from build123d import *

# Parameters (mm, degrees)
SKETCH1_W           = 40.8
SKETCH1_H           = 20
BOSS_EXTRUDE1_DEPTH = 36.4
SKETCH2_W           = 40.8
SKETCH2_H           = 20
SKETCH2_W_2         = 37.24847256
SKETCH2_H_2         = 17
CUT_EXTRUDE1_DEPTH  = 4.6
SKETCH3_W           = 37.24847256
SKETCH3_H           = 17
SKETCH3_R           = 5
CUT_EXTRUDE2_DEPTH  = 3.9
SKETCH4_R           = 5
SKETCH4_R_2         = 3.5
CUT_EXTRUDE3_DEPTH  = 3
FILLET1_R           = 1
FILLET2_R           = 0.25


with BuildPart() as part:
    # Sketch1 → Boss-Extrude1 (new body)
    with BuildSketch(Plane(origin=(0, 0, 0), x_dir=(1, 0, 0), z_dir=(0, 1, 0))):
        Rectangle(SKETCH1_W, SKETCH1_H)
    extrude(amount=BOSS_EXTRUDE1_DEPTH)

    # Sketch2 → Cut-Extrude1 (cut)
    with BuildSketch(Plane(origin=(0, 0, 0), x_dir=(1, 0, 0), z_dir=(0, 1, 0))):
        Rectangle(SKETCH2_W, SKETCH2_H)
        Rectangle(SKETCH2_W_2, SKETCH2_H_2, mode=Mode.SUBTRACT)
    extrude(amount=CUT_EXTRUDE1_DEPTH, mode=Mode.SUBTRACT)

    # Sketch3 → Cut-Extrude2 (cut)
    with BuildSketch(Plane(origin=(0, 0, 0), x_dir=(1, 0, 0), z_dir=(0, 1, 0))):
        Rectangle(SKETCH3_W, SKETCH3_H)
        with Locations((9.31211814, 0)):
            Circle(SKETCH3_R, mode=Mode.SUBTRACT)
    extrude(amount=CUT_EXTRUDE2_DEPTH, mode=Mode.SUBTRACT)

    # Sketch4 → Cut-Extrude3 (cut)
    with BuildSketch(Plane(origin=(0, 0, 0), x_dir=(1, 0, 0), z_dir=(0, 1, 0))):
        with Locations((9.31211814, 0)):
            Circle(SKETCH4_R)
        with Locations((9.31211814, 0)):
            Circle(SKETCH4_R_2, mode=Mode.SUBTRACT)
    extrude(amount=CUT_EXTRUDE3_DEPTH, mode=Mode.SUBTRACT)

    # Fillet1
    fillet1_edges = [part.edges().sort_by_distance(p)[0] for p in [
        (20.4, 36.4, 0),
        (0, 36.4, -10),
        (-20.4, 4.6, 0),
        (0, 4.6, 10),
        (20.4, 4.6, 0),
        (0, 4.6, -10),
        (-20.4, 36.4, 0),
        (0, 36.4, 10),
        (-20.4, 20.5, -10),
        (20.4, 20.5, -10),
        (20.4, 20.5, 10),
        (-20.4, 20.5, 10),
    ]]
    fillet(fillet1_edges, radius=FILLET1_R)

    # Fillet2
    fillet2_edges = [part.edges().sort_by_distance(p)[0] for p in [
        (-18.62423628, 4.6, 0),
        (0, 4.6, 8.5),
        (18.62423628, 4.6, 0),
        (18.62423628, 4.25, -8.5),
        (0, 4.6, -8.5),
        (-18.62423628, 4.25, -8.5),
        (-18.62423628, 3.9, 0),
        (0, 3.9, 8.5),
        (18.62423628, 3.9, 0),
        (0, 3.9, -8.5),
    ]]
    fillet(fillet2_edges, radius=FILLET2_R)


solid = part.part
Here's how the part is built. I have some questions about the finished solid (model axes, mm). A direction names the side the tool comes from. Round coordinates to 2 decimals unless told otherwise and drop trailing zeros. Loops run counter-clockwise (first coordinate to the right, second up) from the corner with the lowest first, then second, coordinate; pieces in that order, holes last.
1. If I drill on line 1 along Y through (x, z) = (-5.5, 2.5); line 2 along Z through (x, y) = (10, 35.5); line 3 along Y through (x, z) = (-17, 9.25), over which ranges is the centre line in solid material (lowest first)?
Answer list:
line 1: y = 3.9 to 36.4
line 2: z = -9.99 to 9.99
line 3: y = 4.63 to 36.37
2. If we section it at A-A on z = 0: Write out the boundary of the cut face in (x, y), plus the area to 3 significant figures.
Answer list:
outline: (-20.4, 5.6) arc R1 ccw to (-19.4, 4.6) - (-18.87, 4.6) arc R0.25 cw to (-18.62, 4.35) - (-18.62, 4.15) arc R0.25 ccw to (-18.37, 3.9) - (4.31, 3.9) - (4.31, 3) - (5.81, 3) - (5.81, 0) - (12.81, 0) - (12.81, 3) - (14.31, 3) - (14.31, 3.9) - (18.37, 3.9) arc R0.25 ccw to (18.62, 4.15) - (18.62, 4.35) arc R0.25 cw to (18.87, 4.6) - (19.4, 4.6) arc R1 ccw to (20.4, 5.6) - (20.4, 35.4) arc R1 ccw to (19.4, 36.4) - (-19.4, 36.4) arc R1 ccw to (-20.4, 35.4) - close
area: 1,350 mm2
3. For P1, Ø5.5, axis at x = -3.5, z = -1, coming from the -Y side, with a flat end and sliding along its axis, tell me the tip position at first contact or that it passes through.
Answer list:
P1: stops at y = 3.9
4. If we section it at B-B on x = -14: Write out the boundary of the cut face in (y, z), plus the area to 3 significant figures.
Answer list:
outline: (3.9, -8.25) arc R0.25 ccw to (4.15, -8.5) - (4.35, -8.5) arc R0.25 cw to (4.6, -8.75) - (4.6, -9) arc R1 ccw to (5.6, -10) - (35.4, -10) arc R1 ccw to (36.4, -9) - (36.4, 9) arc R1 ccw to (35.4, 10) - (5.6, 10) arc R1 ccw to (4.6, 9) - (4.6, 8.75) arc R0.25 cw to (4.35, 8.5) - (4.15, 8.5) arc R0.25 ccw to (3.9, 8.25) - close
area: 647 mm2
5. Which directions (+Z, -Z, +X, -X, +Y, -Y) give clear straight access to the entire face, cutting with the end or side of a thin tool? Please do faces 1 (the face through (13.93, 3.44, 1.92)), 2 (the face through (20.099, 4.885, -0.126)).
Answer list:
face 1: -Y
face 2: +Z, -Z, +X, -Y
6. If we section it at C-C on z = -4.25: Write out the boundary of the cut face in (x, y).
Answer list:
outline: (-20.4, 5.6) arc R1 ccw to (-19.4, 4.6) - (-18.87, 4.6) arc R0.25 cw to (-18.62, 4.35) - (-18.62, 4.15) arc R0.25 ccw to (-18.37, 3.9) - (6.68, 3.9) - (6.68, 3) - (11.95, 3) - (11.95, 3.9) - (18.37, 3.9) arc R0.25 ccw to (18.62, 4.15) - (18.62, 4.35) arc R0.25 cw to (18.87, 4.6) - (19.4, 4.6) arc R1 ccw to (20.4, 5.6) - (20.4, 35.4) arc R1 ccw to (19.4, 36.4) - (-19.4, 36.4) arc R1 ccw to (-20.4, 35.4) - close
